from build123d import *

# Parameters (mm, degrees)
SKETCH1_W           = 112.268
SKETCH1_H           = 101.6
SKETCH1_W_2         = 57.658
SKETCH1_H_2         = 25.908
BOSS_EXTRUDE1_DEPTH = 25.4
SKETCH2_W           = 86.868
SKETCH2_H           = 31.496
CUT_EXTRUDE1_DEPTH  = 80.855030875
SKETCH4_R           = 3.429
CUT_EXTRUDE2_DEPTH  = 94.331435069
SKETCH5_R           = 3.429
CUT_EXTRUDE3_DEPTH  = 80.855030875


with BuildPart() as part:
    # Sketch1 → Boss-Extrude1 (new body)
    with BuildSketch(Plane(origin=(0, 0, 0), x_dir=(1, 0, 0), z_dir=(0, 1, 0))):
        Rectangle(SKETCH1_W, SKETCH1_H)
        Rectangle(SKETCH1_W_2, SKETCH1_H_2, mode=Mode.SUBTRACT)
    extrude(amount=BOSS_EXTRUDE1_DEPTH)

    # Sketch2 → Cut-Extrude1 (cut, through all)
    with BuildSketch(Plane(origin=(0, 0, 0), x_dir=(1, 0, 0), z_dir=(0, 1, 0))):
        with Locations((12.7, 35.052)):
            Rectangle(SKETCH2_W, SKETCH2_H)
    extrude(amount=CUT_EXTRUDE1_DEPTH, mode=Mode.SUBTRACT)

    # Sketch4 → Cut-Extrude2 (cut, through all)
    with BuildSketch(Plane(origin=(0, 0, -19.304), x_dir=(-1, 0, 0), z_dir=(0, 0, -1))):
        with Locations((-22.225, 12.190161911)):
            Circle(SKETCH4_R)
        with Locations((22.225, 12.190161911)):
            Circle(SKETCH4_R)
    extrude(amount=-CUT_EXTRUDE2_DEPTH, mode=Mode.SUBTRACT)

    # Sketch5 → Cut-Extrude3 (cut, through all)
    with BuildSketch(Plane(origin=(0, 25.4, 0), x_dir=(1, 0, 0), z_dir=(0, 1, 0))):
        with Locations(Location((-43.434, 25.4, 0), (0, 0, 270))):
            Circle(SKETCH5_R)
        with Locations(Location((-43.434, -25.4, 0), (0, 0, 270))):
            Circle(SKETCH5_R)
    extrude(amount=-CUT_EXTRUDE3_DEPTH, mode=Mode.SUBTRACT)


solid = part.part
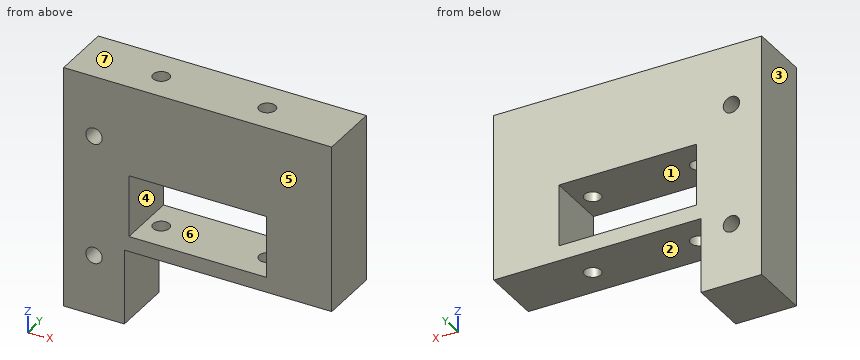
The model under review builds one solid part; all positions refer to its coordinate system, in mm. Face numbers are marked on the shaded views. A direction names the side the tool comes from. Coordinates: 2 decimals unless noted, no trailing zeros. Write each loop counter-clockwise with the first axis right and the second up, starting at its lowest first coordinate (ties: lowest second). Pieces come first, ordered by that corner, then holes. Notation, with made-up numbers: M 44,45.5 L 57,45.5 A27 cw 57,77.5 Z; hole C -26,16 d7. An arc over 180 degrees is marked long. Put each result on its own line as item: value.
1) For the marked faces 1, 2 and 3, list the 3-axis set-ups (+Z, -Z, +X, -X, +Y, -Y) from which the entire face can be reached by the end or side of a thin tool; tool diameter is ignored.
Computed:
face 1: +Y, -Y
face 2: -Z, +X, +Y, -Y
face 3: +Z, -Z, -X, +Y, -Y
2) Add section A-A on z = 25.4. Give the boundary of the cut face in (x, y) (3 decimals).
Computed:
outline: M -56.134,0 L -46.863,0 L -46.863,25.4 L -56.134,25.4 Z; M -40.005,0 L 56.134,0 L 56.134,25.4 L -40.005,25.4 Z; hole C -22.225,12.19 d6.858; hole C 22.225,12.19 d6.858
3) Add section C-C on y = 17.75. Give the boundary of the cut face in (x, z), then the cut area to 3 significant figures.
Computed:
outline: M -56.13,-50.8 L -30.73,-50.8 L -30.73,-19.3 L 56.13,-19.3 L 56.13,50.8 L -56.13,50.8 Z; hole C -43.43,-25.4 d6.86; hole C -43.43,25.4 d6.86; hole M -28.83,-12.95 L 28.83,-12.95 L 28.83,12.95 L -28.83,12.95 Z
area: 7,100 mm2
4) Wall thickness on probe 1 along X at (y, z) = (18.5, 25.4) (3 decimals); probe 2 along X at (y, z) = (6.25, -7); probe 3 along Z at (x, y) = (-21, 24.75): over which ranges is each line inside the solid? List them lowest first. Write a range as [from, to].
Computed:
probe 1: x = [-56.134, -46.863], [-40.005, 56.134]
probe 2: x = [-56.13, -28.83], [28.83, 56.13]
probe 3: z = [-19.3, -12.95], [12.95, 50.8]
5) Draft analysis for pull direction Z (two halves, no side actions). For the marked faces 4, 5, 6 and 7, state which applies: released by +Z, released by -Z, zero draft, split by the parting line, or undercut.
Computed:
face 4: undercut
face 5: zero draft
face 6: undercut
face 7: released by +Z
6) Add section B-B on z = -4. Give the boundary of the cut face in (x, y).
Computed:
outline: M -56.13,0 L -28.83,0 L -28.83,25.4 L -56.13,25.4 Z; M 28.83,0 L 56.13,0 L 56.13,25.4 L 28.83,25.4 Z
7) Clearance check with flat-ended pins moving along their axes: pin 1 Ø7.5 at (y, z) = (7.5, -41.5) entering from +X; pin 2 Ø5.5 at (x, y) = (22.22, 12.19) entering from +Z; pin 3 Ø12.5 at (x, y) = (-9.5, 11) entering from -Z. State where each tip first meets the part, or that it passes through.
Computed:
pin 1: stops at x = -30.73
pin 2: passes through
pin 3: stops at z = -19.3
8) Add section D-D on x = 40. Give the boundary of the cut face in (y, z).
Computed:
outline: M 0,-19.3 L 25.4,-19.3 L 25.4,50.8 L 0,50.8 Z
